```python
from build123d import *

# Parameters (mm, degrees)
SKETCH_R      = 6
SKETCH_R_2    = 2.5
PAD_DEPTH     = 20.5
SKETCH001_W   = 5.557975
SKETCH001_H   = 5.932069
SKETCH001_W_2 = 3
SKETCH001_H_2 = 5
PAD001_DEPTH  = 20.5
SKETCH003_R   = 7
SKETCH003_R_2 = 2.5
PAD002_DEPTH  = 1
SKETCH004_R   = 7
SKETCH004_R_2 = 2.5
PAD003_DEPTH  = 0.5


with BuildPart() as part:
    # Sketch → Pad (new body)
    with BuildSketch(Plane.XY):
        Circle(SKETCH_R)
        Circle(SKETCH_R_2, mode=Mode.SUBTRACT)
    extrude(amount=PAD_DEPTH)

    # Sketch001 → Pad001 (join)
    with BuildSketch(Plane.XY):
        with Locations((0.008437, -0.106321)):
            Rectangle(SKETCH001_W, SKETCH001_H)
        Rectangle(SKETCH001_W_2, SKETCH001_H_2, mode=Mode.SUBTRACT)
    extrude(amount=PAD001_DEPTH)

    # Sketch003 (on Face5 of Pad001) → Pad002 (join)
    with BuildSketch(Plane.XY.offset(20.5)):
        Circle(SKETCH003_R)
        Circle(SKETCH003_R_2, mode=Mode.SUBTRACT)
    extrude(amount=PAD002_DEPTH)

    # Sketch004 → Pad003 (join, symmetric)
    with BuildSketch(Plane.XY):
        Circle(SKETCH004_R)
        Circle(SKETCH004_R_2, mode=Mode.SUBTRACT)
    extrude(amount=PAD003_DEPTH, both=True)


solid = part.part
```
Model file for the job. Use its own axes, mm. A direction names the side the tool comes from. Give positions to 0.01 mm unless a question says otherwise; leave off trailing zeros. Loops run counter-clockwise (first coordinate to the right, second up) from the corner with the lowest first, then second, coordinate; pieces in that order, holes last. Notation, with made-up numbers: (45.25, 86) - (75.25, 86) arc R18 cw to (75.25, 94) - close; hole circle Ø5 at (-22, 85). An arc over 180 degrees is marked (long way). One line per item, written item: value. Start each with the question number.
1. Slice it at B-B (x = 0). List the corners of the cut face in (y, z), plus the area to 3 significant figures.
2. Which spindle directions (+Z, -Z, +X, -X, +Y, -Y) get a long thin tool onto all of the face, cutting with end or side? Do faces 4 (the flat face through (2, 0, 0)), 5 (the flat face through (6, 2, 20.5)), 6 (the flat face through (-2, 0, 20.5)). Say none if no direction does.
3. Probe L1, parallel to Y at x = 0, z = 15.5; L2, parallel to X at y = 0, z = 15; L3, parallel to Y at x = -1, z = 7.25. List the from-to ranges inside material, lowest first. Write a range as from..to.
4. Pull direction X, two halves, no side cores. Call faces 1 (the flat face through (0, -3, 21.5)), 2 (the flat face through (-1.5, 0, 10)), 3 (the cylindrical face through (-6, 0, 10)): pulls with the +X half, pulls with the -X half, needs draft (parallel to the pull), parting line crosses it, or undercut.
5. Pin check, flat tips, straight feed: pin 1 (6 mm diameter, centred on x = -2.5, z = 8.5, fed in from +Y); pin 2 (5 mm diameter, centred on x = 0, z = 2.5, fed in from +Y); pin 3 (1 mm diameter, centred on y = -4, z = 4.5, fed in from -X); pin 4 (2 mm diameter, centred on y = 0, z = 15, fed in from -X). Stop position of each tip, or through.
6. Slice it at D-D (y = 5.75). List the corners of the cut face in (x, z), plus the area to 3 significant figures.
7. Slice it at C-C (z = 3.5). List the corners of the cut face in (x, y).
8. Slice it at A-A (y = 0). List the corners of the cut face in (x, z).
Solution:
1. outline: (-7, -0.5) - (-2.5, -0.5) - (-2.5, 21.5) - (-7, 21.5) - (-7, 20.5) - (-6, 20.5) - (-6, 0.5) - (-7, 0.5) - close; (2.5, -0.5) - (7, -0.5) - (7, 0.5) - (6, 0.5) - (6, 20.5) - (7, 20.5) - (7, 21.5) - (2.5, 21.5) - close
1. area: 158 mm^2
2. face 4: -Z
2. face 5: none
2. face 6: +Z
3. L1: y = -6..-2.5, 2.5..6
3. L2: x = -6..-1.5, 1.5..6
3. L3: y = -5.92..-2.29, 2.29..5.92
4. face 1: needs draft
4. face 2: undercut
4. face 3: parting line crosses it
5. pin 1: stops at y = 6
5. pin 2: stops at y = 7
5. pin 3: stops at x = -4.87
5. pin 4: stops at x = -6
6. outline: (-3.99, -0.5) - (3.99, -0.5) - (3.99, 0.5) - (1.71, 0.5) - (1.71, 20.5) - (3.99, 20.5) - (3.99, 21.5) - (-3.99, 21.5) - (-3.99, 20.5) - (-1.71, 20.5) - (-1.71, 0.5) - (-3.99, 0.5) - close
6. area: 84.5 mm^2
7. outline: circle Ø12 at (0, 0); hole (-1.5, -2) arc R2.5 ccw to (1.5, -2) - (1.5, 2) arc R2.5 ccw to (-1.5, 2) - close
8. outline: (-7, -0.5) - (-2.5, -0.5) - (-2.5, 0) - (-1.5, 0) - (-1.5, 20.5) - (-2.5, 20.5) - (-2.5, 21.5) - (-7, 21.5) - (-7, 20.5) - (-6, 20.5) - (-6, 0.5) - (-7, 0.5) - close; (1.5, 0) - (2.5, 0) - (2.5, -0.5) - (7, -0.5) - (7, 0.5) - (6, 0.5) - (6, 20.5) - (7, 20.5) - (7, 21.5) - (2.5, 21.5) - (2.5, 20.5) - (1.5, 20.5) - close
